from build123d import *

# Parameters (mm, degrees)
F1_DEPTH = 6.35
F4_R     = 11.176
F5_DEPTH = 25.4
F6_R     = 12.7
F7_R     = 11.176
F8_DEPTH = 25.4


# Not quite as in the source:
# - a feature of the source that left no trace in its solid (it failed there, or was rolled back) is left out


with BuildPart() as f1:
    # F0 (on Front) → F1 (new body)
    with BuildSketch(Plane.XZ):
        with BuildLine():
            Line((19.9482194655, 24.7153370319), (0, 59.2666666667))
            Line((0, 59.2666666667), (-19.9482194655, 24.7153370319))
            ThreePointArc((-19.9482194655, 24.7153370319), (-15.7645491002, 20.5316666667), (-14.2332194655, 14.8166666667))
            ThreePointArc((-14.2332194655, 14.8166666667), (-19.9482194655, 4.9179963014), (-31.3782194655, 4.9179963014))
            Line((-31.3782194655, 4.9179963014), (-51.326438931, -29.6333333333))
            Line((-51.326438931, -29.6333333333), (-11.43, -29.6333333333))
            ThreePointArc((-11.43, -29.6333333333), (0, -18.2033333333), (11.43, -29.6333333333))
            Line((11.43, -29.6333333333), (51.326438931, -29.6333333333))
            Line((51.326438931, -29.6333333333), (31.3782194655, 4.9179963014))
            ThreePointArc((31.3782194655, 4.9179963014), (15.7645491002, 9.1016666667), (19.9482194655, 24.7153370319))
        make_face()
    extrude(amount=F1_DEPTH)

    # F4 (on face) → F5 (cut)
    with BuildSketch(Plane(origin=(0, 0, 0), x_dir=(-1, 0, 0), z_dir=(0, 1, 0))):
        with Locations((0, 28.7866666667)):
            Circle(F4_R)
        with Locations((-25.0159751206, -14.245354451)):
            Circle(F4_R)
        with Locations((24.9412614338, -14.3738179923)):
            Circle(F4_R)
    extrude(amount=-F5_DEPTH, mode=Mode.SUBTRACT)

    # F6
    f6_edges = [f1.edges().sort_by_distance(p)[0] for p in [
        (0, -3.175, 59.266667),
        (51.326439, -3.175, -29.633333),
        (-51.326439, -3.175, -29.633333),
    ]]
    fillet(f6_edges, radius=F6_R)

    # F7 (on face) → F8 (cut)
    with BuildSketch(Plane(origin=(0, 0, 0), x_dir=(-1, 0, 0), z_dir=(0, 1, 0))):
        Circle(F7_R)
    extrude(amount=-F8_DEPTH, mode=Mode.SUBTRACT)


solid = f1.part
Could you check a few things on this model? Use its own coordinates, in mm. Give positions to 0.01 mm unless a question says otherwise; leave off trailing zeros. Order: outer loops, then holes, each group sorted by start corner. A loop starts at its lowest first (then second) coordinate and runs counter-clockwise, first axis right, second up.
1. Suppose I cut it at C-C (y = -1.25). List the corners of the cut face in (x, z) for me, plus the area to 3 significant figures.
2. Suppose I cut it at D-D (x = 33). List the corners of the cut face in (y, z) for me.
3. We'd pull the mould along X, two halves only. Please class faces 1 (the cylindrical face through (36.18, -3.13, -13.75)), 2 (the flat face through (-15.411, -3.131, 32.575)), 3 (the cylindrical face through (0.186, -3.219, 46.565)), 4 (the flat face through (3, 0, -11)): pulls with the +X half, pulls with the -X half, needs draft (parallel to the pull), parting line crosses it, or undercut.
4. Suppose I cut it at A-A (x = 0). List the corners of the cut face in (y, z) for me.
5. Will these pins go through, and if not, where does the flat tip stop? P1, Ø3, axis at x = -9, y = -1, coming from the +Z side; P2, Ø1, axis at y = -1, z = -5, coming from the -X side; P3, Ø3, axis at x = -8, y = -5.5, coming from the +Z side.
6. I need wall thicknesses on L1, parallel to X at y = -2.75, z = -7.5; L2, parallel to X at y = -3.75, z = -4.5; L3, parallel to X at y = -1, z = -17.5. Which ranges of each line are inside material? Lowest first, please.
7. Suppose I cut it at B-B (z = -7). List the corners of the cut face in (x, y) for me.
Solved:
1. outline: (-40.33, -10.58) arc R12.7 ccw to (-29.33, -29.63) - (-11.43, -29.63) arc R11.43 cw to (11.43, -29.63) - (29.33, -29.63) arc R12.7 ccw to (40.33, -10.58) - (31.38, 4.92) arc R11.43 cw to (19.95, 24.72) - (11, 40.22) arc R12.7 ccw to (-11, 40.22) - (-19.95, 24.72) arc R11.43 cw to (-31.38, 4.92) - close; hole circle Ø22.35 at (-24.94, -14.37); hole circle Ø22.35 at (0, 0); hole circle Ø22.35 at (0, 28.79); hole circle Ø22.35 at (25.02, -14.25)
1. area: 2,050 mm2
2. outline: (-6.35, -29.09) - (0, -29.09) - (0, -22.07) - (-6.35, -22.07) - close; (-6.35, -6.42) - (0, -6.42) - (0, 2.11) - (-6.35, 2.11) - close
3. face 1: undercut
3. face 2: pulls with the -X half
3. face 3: parting line crosses it
3. face 4: needs draft
4. outline: (-6.35, -18.2) - (0, -18.2) - (0, -11.18) - (-6.35, -11.18) - close; (-6.35, 11.18) - (0, 11.18) - (0, 17.61) - (-6.35, 17.61) - close; (-6.35, 39.96) - (0, 39.96) - (0, 46.57) - (-6.35, 46.57) - close
5. P1: stops at z = 44.12
5. P2: stops at x = -37.39
5. P3: stops at z = 44.78
6. L1: x = -38.55 to -33.75, -16.13 to -8.29, 8.29 to 16.11, 33.93 to 38.55
6. L2: x = -36.82 to -30.18, -19.71 to -10.23, 10.23 to 19.55, 30.49 to 36.82
6. L3: x = -42.02 to -35.67, -14.21 to 14.32, 35.71 to 42.02
7. outline: (-38.26, -6.35) - (-33.34, -6.35) - (-33.34, 0) - (-38.26, 0) - close; (-16.54, -6.35) - (-8.71, -6.35) - (-8.71, 0) - (-16.54, 0) - close; (8.71, -6.35) - (16.51, -6.35) - (16.51, 0) - (8.71, 0) - close; (33.53, -6.35) - (38.26, -6.35) - (38.26, 0) - (33.53, 0) - close
